Verification items for this drawing (mm, ordinates from the low corner). A direction names the side the tool comes from. Round coordinates to 2 decimals unless told otherwise and drop trailing zeros. Order: outer loops, then holes, each group sorted by start corner. A loop starts at its lowest first (then second) coordinate and runs counter-clockwise, first axis right, second up. Notation, with made-up numbers: (20, -36.75) - (33, -36.75) arc R22 ccw to (33, -27.75) - close; hole circle Ø8 at (55.5, -4). An arc over 180 degrees is marked (long way). Return JSON: item names as keys, results as strings. Group by question number.
Q1. Sectioned sample at A-A, the plane z = 15. Record the cut outline in (x, y).
Q2. Gauge pin test, flat ends, axial feed: pin 1 Ø6 at (x, y) = (29.5, 14) entering from +Z; pin 2 Ø1.5 at (x, z) = (36.5, 16) entering from -Y. Record the tip position at first contact, or that the pin passes through.
Q3. Sectioned sample at C-C, the plane y = 93. Record the cut outline in (x, z), then the cut area to 3 significant figures.
Q4. Material ranges on line 1 along X through (y, z) = (59, 4); line 2 along Y through (x, z) = (40.5, 16.75); line 3 along Z through (x, y) = (77.5, 69), recorded low to high.
Q5. Sectioned sample at B-B, the plane x = 91.5. Record the cut outline in (y, z).
Q6. Tool access check on the marked faces 4 and 5. Record the directions out of +Z, -Z, +X, -X, +Y, -Y that give a thin tool (end or side, any length) a straight path to the whole face; none if there is none.
Q7. Draft check along X on the marked faces 1, 2 and 3. Enter one of: pulls with the +X half, pulls with the -X half, needs draft (parallel to the pull), parting line crosses it, or undercut.
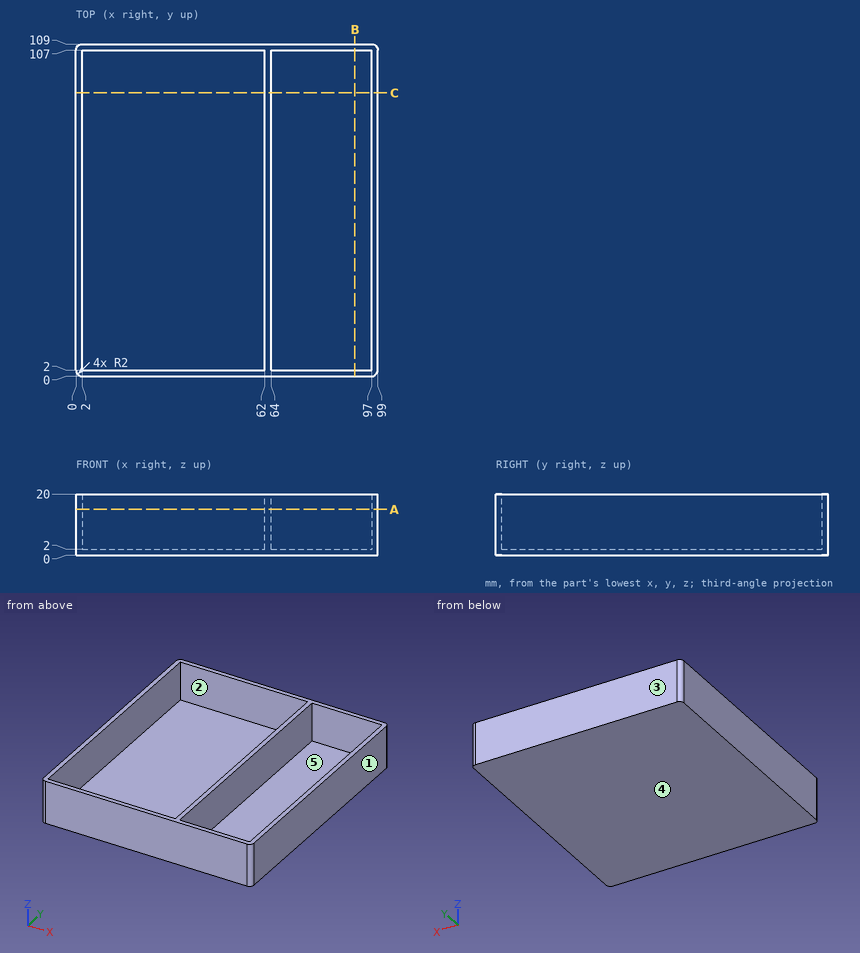
Reply:
{
 "1": {"outline": "(0, 2) arc R2 ccw to (2, 0) - (97, 0) arc R2 ccw to (99, 2) - (99, 107) arc R2 ccw to (97, 109) - (2, 109) arc R2 ccw to (0, 107) - close; hole (2, 2) - (62, 2) - (62, 107) - (2, 107) - close; hole (64, 2) - (97, 2) - (97, 107) - (64, 107) - close"},
 "2": {"pin 1": "z = 2", "pin 2": "y = 0"},
 "3": {"outline": "(0, 0) - (99, 0) - (99, 20) - (97, 20) - (97, 2) - (64, 2) - (64, 20) - (62, 20) - (62, 2) - (2, 2) - (2, 20) - (0, 20) - close", "area": "306 mm^2"},
 "4": {"line 1": "0 to 2, 62 to 64, 97 to 99", "line 2": "0 to 2, 107 to 109", "line 3": "0 to 2"},
 "5": {"outline": "(0, 0) - (109, 0) - (109, 20) - (107, 20) - (107, 2) - (2, 2) - (2, 20) - (0, 20) - close"},
 "6": {"face 4": "-Z, +X, -X, +Y, -Y", "face 5": "+Z"},
 "7": {"face 1": "pulls with the +X half", "face 2": "undercut", "face 3": "needs draft"}
}
